```python
from build123d import *

# Parameters (mm, degrees)
BOSS_EXTRUDE1_DEPTH      = 3.75
BOSS_EXTRUDE1_DEPTH_BACK = 3.75
SKETCH1_R                = 9.635
SKETCH1_R_2              = 7.635
FILLET1_R                = 0.7
FILLET3_R                = 0.7
CUT_REVOLVE2_START       = -3.05
CUT_REVOLVE2_DEPTH       = 6.1


# Read off the part's stored shape, not the designer's step: Cut-Revolve2
with BuildPart() as part:
    # Sketch1 → Boss-Extrude1 (new, two sides: drawn at the far end of the back side and taken through both)
    with BuildSketch(Plane(origin=(0, 0, 0), x_dir=(1, 0, 0), z_dir=(0, 1, 0)).offset(-BOSS_EXTRUDE1_DEPTH_BACK)):
        with Locations(Location((0, 0, 0), (0, 0, 270))):
            Circle(SKETCH1_R)
        with Locations(Location((0, 0, 0), (0, 0, 270))):
            Circle(SKETCH1_R_2, mode=Mode.SUBTRACT)
    extrude(amount=BOSS_EXTRUDE1_DEPTH + BOSS_EXTRUDE1_DEPTH_BACK)

    # Fillet1
    fillet1_edges = [part.edges().sort_by_distance(p)[0] for p in [
        (0, -3.75, -9.635),
        (0, 3.75, -9.635),
    ]]
    fillet(fillet1_edges, radius=FILLET1_R)

    # Sketch3 → Cut-Revolve1 (revolve, cut)
    with BuildSketch(Plane(origin=(0, 0, 0), x_dir=(0, 0, -1), z_dir=(1, 0, 0)), mode=Mode.PRIVATE) as cut_revolve1_sk:
        with BuildLine():
            Line((-7.635, 3.75), (-7.635, 0.005))
            ThreePointArc((-7.635, 0.005), (-7.766616425, 1.893305551), (-8.135, 3.75))
            Line((-8.135, 3.75), (-7.635, 3.75))
        make_face()
        with BuildLine():
            Line((-7.635, -3.75), (-8.135, -3.75))
            ThreePointArc((-8.135, -3.75), (-7.766616425, -1.893305551), (-7.635, -0.005))
            Line((-7.635, -0.005), (-7.635, -3.75))
        make_face()
    revolve(cut_revolve1_sk.sketch.rotate(Axis((0, 0, 0), (0, 1, 0)), 180), axis=Axis((0, 0, 0), (0, 1, 0)), mode=Mode.SUBTRACT)

    # Fillet3
    fillet3_edges = [part.edges().sort_by_distance(p)[0] for p in [
        (0, 3.75, 8.135),
        (0, -3.75, 8.135),
    ]]
    fillet(fillet3_edges, radius=FILLET3_R)

    # Cut-Revolve2 outline → Cut-Revolve2 (cut)
    with BuildSketch(Plane(origin=(0, 0, 0), x_dir=(1, 0, 0), z_dir=(0, 1, 0)).offset(CUT_REVOLVE2_START)):
        with BuildLine():
            ThreePointArc((-7.543281251, 3.545579355), (0, 8.335), (7.543281251, 3.545579355))
            Line((7.543281251, 3.545579355), (8.719797823, 4.098579135))
            ThreePointArc((8.719797823, 4.098579135), (0, 9.635), (-8.719797823, 4.098579135))
            Line((-8.719797823, 4.098579135), (-7.543281251, 3.545579355))
        make_face()
    cut_revolve2 = extrude(amount=CUT_REVOLVE2_DEPTH, mode=Mode.SUBTRACT)

    # Mirror3: Cut-Revolve2 across plane
    add(cut_revolve2.mirror(Plane.XY), mode=Mode.SUBTRACT)


solid = part.part
```
Part model, mm, in its own coordinate system. A direction names the side the tool comes from. Round coordinates to 2 decimals unless told otherwise and drop trailing zeros. Loops run counter-clockwise (first coordinate to the right, second up) from the corner with the lowest first, then second, coordinate; pieces in that order, holes last.
1. Slice it at B-B (y = -2.5). Give the cut face in (x, z) (3 decimals), and give its area (3 significant figures).
Solutions:
outline: (-8.72, -4.099) - (-7.543, -3.546) arc R8.335 ccw to (7.543, -3.546) - (8.72, -4.099) arc R9.635 ccw to (8.72, 4.099) - (7.543, 3.546) arc R8.335 ccw to (-7.543, 3.546) - (-8.72, 4.099) arc R9.635 ccw to start; hole circle Ø15.721 at (0, 0)
area: 44.7 mm2
2. Flat gauge pins, fed straight in: pin 1 (3 mm diameter, centred on x = 0.5, z = 7.5, fed in from +Y); pin 2 (3 mm diameter, centred on y = -2, z = 4, fed in from -X) (3 decimals); pin 3 (2 mm diameter, centred on x = -6, y = 2.5, fed in from +Z); pin 4 (3 mm diameter, centred on x = -4, z = -5.5, fed in from -Y). Where does each tip first touch, or does it go through?
Solutions:
pin 1: stops at y = 3.75
pin 2: stops at x = -9.305
pin 3: stops at z = 8.13
pin 4: stops at y = -3.64
3. Two-plate mould, pull along X, no slides. Class faces 1 (the face through (9.635, -0.043, 0.059)), 2 (the face through (-9.635, -0.043, -0.059)), 3 (the face through (-8.14, -0.043, 3.826)): pulls with the +X half, pulls with the -X half, needs draft (parallel to the pull), parting line crosses it, or undercut.
Solutions:
face 1: pulls with the +X half
face 2: pulls with the -X half
face 3: undercut
4. Drill centre lines: line 1 along X through (y, z) = (0, -1.5); line 2 along Z through (x, y) = (-1.5, -3); line 3 along X through (y, z) = (2.25, -7). Where is each one in solid material? Low to high.
Solutions:
line 1: x = -9.52 to -7.49, 7.49 to 9.52
line 2: z = -8.2 to -7.81, 7.81 to 8.2
line 3: x = -4.52 to -3.48, 3.48 to 4.52
5. 3-axis set-ups, long thin cutter, end or side, ignore diameter. For faces 4 (the face through (0, -3.05, 9)), 5 (the face through (8.123, -0.043, -3.818)): which of +Z, -Z, +X, -X, +Y, -Y reach the whole face in a straight line?
Solutions:
face 4: +Z
face 5: -Z
6. Slice it at A-A (y = -1.5). Give the cut face in (x, z) (3 decimals).
Solutions:
outline: (-8.72, -4.099) - (-7.543, -3.546) arc R8.335 ccw to (7.543, -3.546) - (8.72, -4.099) arc R9.635 ccw to (8.72, 4.099) - (7.543, 3.546) arc R8.335 ccw to (-7.543, 3.546) - (-8.72, 4.099) arc R9.635 ccw to start; hole circle Ø15.439 at (0, 0)
